Verification items for this drawing (mm, ordinates from the low corner). A direction names the side the tool comes from. Coordinates: 2 decimals unless noted, no trailing zeros. Write each loop counter-clockwise with the first axis right and the second up, starting at its lowest first coordinate (ties: lowest second). Pieces come first, ordered by that corner, then holes. Notation, with made-up numbers: (39, 19) -> (62, 19) arc R9 ccw to (62, 25) -> close; hole circle Ø6 at (41.25, 72). An arc over 180 degrees is marked (long way). Answer as CSV lines item,"result".
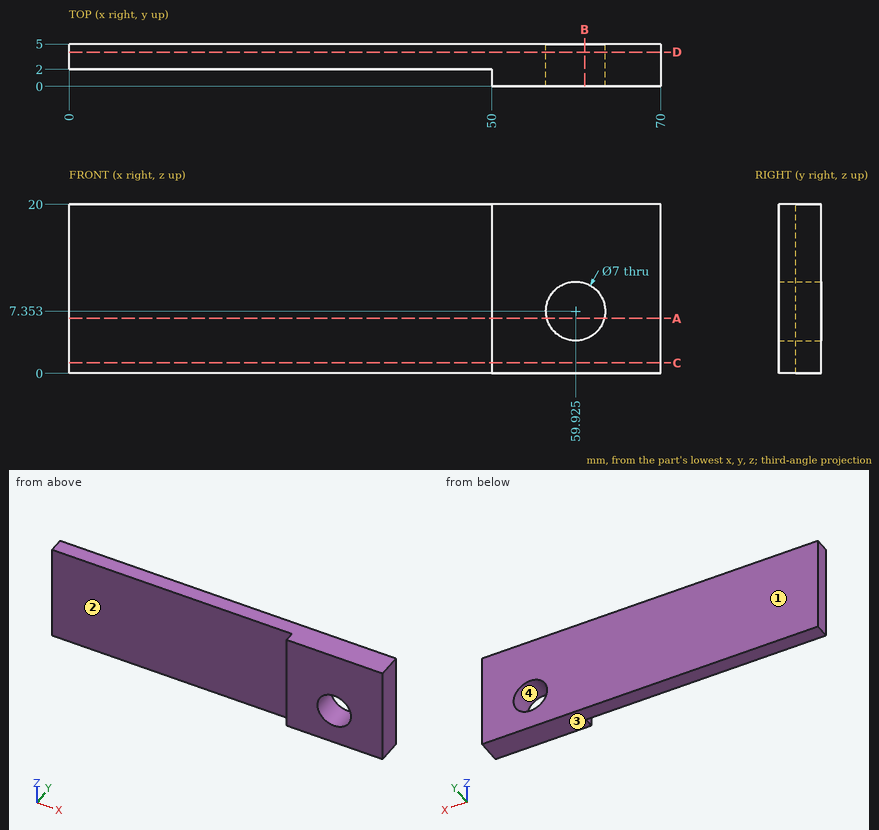
Item 1: Set-up check for the marked faces 1 and 2: record each of +Z, -Z, +X, -X, +Y, -Y from which the full face is reachable in a straight line by a thin tool's end or side.
Responses:
face 1,"+Z, -Z, +X, -X, +Y"
face 2,"+Z, -Z, -X, -Y"
Item 2: Thickness scan on probe 1 along Z at (x, y) = (60, 1.25); probe 2 along Y at (x, z) = (46.5, 2.5); probe 3 along X at (y, z) = (0.5, 17). Record the ranges inside material, lowest first.
Responses:
probe 1,"z = 0 to 3.85, 10.85 to 20"
probe 2,"y = 2 to 5"
probe 3,"x = 50 to 70"
Item 3: Cross-section at D-D, the plane y = 4.05. Record the cut outline in (x, z) (3 decimals).
Responses:
outline,"(0, 0) -> (70, 0) -> (70, 20) -> (0, 20) -> close; hole circle Ø7 at (59.925, 7.353)"
Item 4: Release check for a two-part mould opening along X. For the marked faces 3 and 4 record: +X half, -X half, draft (parallel to the pull), parting line (faces both ways), or undercut.
Responses:
face 3,"draft"
face 4,"undercut"
Item 5: Cross-section at A-A, the plane z = 6.5. Record the cut outline in (x, y).
Responses:
outline,"(0, 2) -> (50, 2) -> (50, 0) -> (56.53, 0) -> (56.53, 5) -> (0, 5) -> close; (63.32, 0) -> (70, 0) -> (70, 5) -> (63.32, 5) -> close"
Item 6: Cross-section at B-B, the plane x = 61. Record the cut outline in (y, z).
Responses:
outline,"(0, 0) -> (5, 0) -> (5, 4.02) -> (0, 4.02) -> close; (0, 10.68) -> (5, 10.68) -> (5, 20) -> (0, 20) -> close"
Item 7: Cross-section at C-C, the plane z = 1.25. Record the cut outline in (x, y).
Responses:
outline,"(0, 2) -> (50, 2) -> (50, 0) -> (70, 0) -> (70, 5) -> (0, 5) -> close"
Item 8: Depth check by flat-ended pin: pin 1 Ø10 at (x, z) = (28, 8.5) entering from -Y; pin 2 Ø3 at (x, y) = (24.5, 4) entering from -Z; pin 3 Ø0.6 at (y, z) = (1, 11.5) entering from -X. Enter the tip coordinate at first touch or a pass-through.
Responses:
pin 1,"stops at y = 2"
pin 2,"stops at z = 0"
pin 3,"stops at x = 50"
